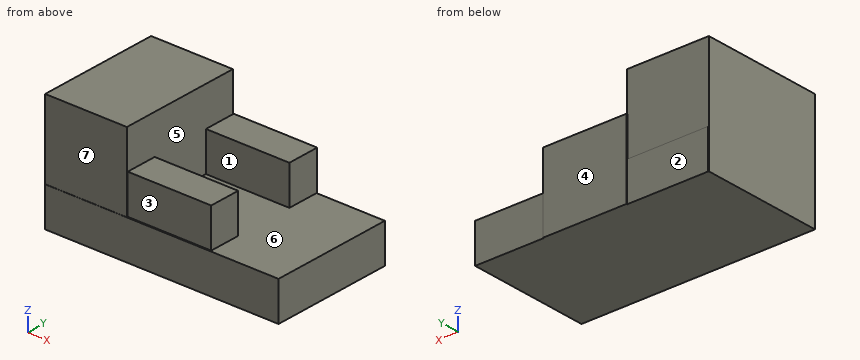
```python
from build123d import *

# Parameters (mm, degrees)
F0_W     = 152.754978
F0_H     = 80.941722
F1_DEPTH = 25.4
F2_W     = 53.560414
F2_H     = 80.67124
F3_DEPTH = 76.2
F4_W     = 54.882895
F4_H     = 20.498429
F4_H_2   = 21.159672
F5_DEPTH = 50.8


with BuildPart() as f1:
    # F0 (on Top) → F1 (new body)
    with BuildSketch(Plane.XY):
        Rectangle(F0_W, F0_H)
    extrude(amount=F1_DEPTH)

    # F2 (on Top) → F3 (join)
    with BuildSketch(Plane.XY):
        with Locations((-49.923595, -2e-06)):
            Rectangle(F2_W, F2_H)
    extrude(amount=F3_DEPTH)

    # F4 (on Top) → F5 (join)
    with BuildSketch(Plane.XY):
        with Locations((4.134902, -29.425164)):
            Rectangle(F4_W, F4_H)
        with Locations((4.134902, 30.417025)):
            Rectangle(F4_W, F4_H_2)
    extrude(amount=F5_DEPTH)


solid = f1.part
```
Work out the finished part from the listing and answer in its coordinate system (mm). Face numbers are marked on the shaded views. A direction names the side the tool comes from. Give positions to 0.01 mm unless a question says otherwise; leave off trailing zeros. Loops run counter-clockwise (first coordinate to the right, second up) from the corner with the lowest first, then second, coordinate; pieces in that order, holes last. Notation, with made-up numbers: M 18.5,24 L 43.5,24 A13 cw 43.5,43 Z; hole C -7,16.5 d2. An arc over 180 degrees is marked long. One line per item, written item: value. Start each with the question number.
1. Which of the six approach directions +Z, -Z, +X, -X, +Y, -Y give full straight-line access (tool end or side, diameter ignored) to the marked faces 1, 2 and 3?
2. Find section D-D (y = 26). Give the vertices of the cut face in (x, z), and give its area (3 significant figures).
3. Find the intervals of material crossed by probe 1 along Z at (x, y) = (46.5, -22.5); probe 2 along Y at (x, z) = (-52, 42); probe 3 along X at (y, z) = (4.5, 71), in increasing order.
4. Find section B-B (z = 49). Give the vertices of the cut face in (x, y).
5. Each of these flat-tipped pins is pushed along its axis until it touches: P1, Ø4, axis at x = -50.5, z = 45.5, coming from the +Y side; P2, Ø10, axis at x = -4, y = -26, coming from the +Z side; P3, Ø16.5, axis at y = -31, z = 36.5, coming from the +X side. Where does it stop, or does it pass through?
6. Determine the mould class of the marked faces 4, 5, 6 and 7 for opening direction Y: released by +Y, released by -Y, zero draft, split by the parting line, or undercut.
7. Find section A-A (x = 15). Give the vertices of the cut face in (y, z), and give its area (3 significant figures).
8. Find section C-C (y = -7). Give the vertices of the cut face in (x, z).
Reported:
1. face 1: +Z, +X
1. face 2: +Z, -Z, -X, +Y
1. face 3: +Z, +X, -Y
2. outline: M -76.7,0 L 76.38,0 L 76.38,25.4 L 31.58,25.4 L 31.58,50.8 L -23.14,50.8 L -23.14,76.2 L -76.7,76.2 Z
2. area: 8,000 mm²
3. probe 1: z = 0 to 25.4
3. probe 2: y = -40.34 to 40.34
3. probe 3: x = -76.7 to -23.14
4. outline: M -76.7,-40.34 L -23.14,-40.34 L -23.14,-39.67 L 31.58,-39.67 L 31.58,-19.18 L -23.14,-19.18 L -23.14,19.84 L 31.58,19.84 L 31.58,41 L -23.31,41 L -23.31,40.34 L -76.7,40.34 Z
5. P1: stops at y = 40.34
5. P2: stops at z = 50.8
5. P3: stops at x = 31.58
6. face 4: released by +Y
6. face 5: undercut
6. face 6: undercut
6. face 7: released by -Y
7. outline: M -40.47,0 L 41,0 L 41,50.8 L 19.84,50.8 L 19.84,25.4 L -19.18,25.4 L -19.18,50.8 L -39.67,50.8 L -39.67,25.4 L -40.47,25.4 Z
7. area: 3,130 mm²
8. outline: M -76.7,0 L 76.38,0 L 76.38,25.4 L -23.14,25.4 L -23.14,76.2 L -76.7,76.2 Z
